Read the model definition and answer for the solid it produces. Units are mm, in the model's axes. A direction names the side the tool comes from. Give positions to 0.01 mm unless a question says otherwise; leave off trailing zeros. Order: outer loops, then holes, each group sorted by start corner. A loop starts at its lowest first (then second) coordinate and runs counter-clockwise, first axis right, second up. Notation, with made-up numbers: (-5.5, 68.25) -> (6.5, 68.25) arc R29 cw to (6.5, 93.25) -> close; hole circle Ø7 at (10, 75.5). An arc over 180 degrees is marked (long way). Answer as CSV lines item,"result". Start each with the question number.
1) A straight line is drawn through the part: L1, parallel to X at y = 212.5, z = 26. Find the intervals that lie inside material, in ascending order. Write a range as from..to.
2) Find section A-A (x = 60.5). Determine the outline of the cut face in (y, z).
3) Find section C-C (z = 13.5). Determine the outline of the cut face in (x, y).
4) For faces 1 (the face through (490, 252, 25)), 2 (the face through (247, 500, 25)), determine the directions among +Z, -Z, +X, -X, +Y, -Y from which every point of the face is accessible in a straight line to the end or side of a thin tool.
5) The mould has two halves that part along Y. Classify faces 3 (the face through (253, 0, 25)), 4 (the face through (10, 258, 25)), 5 (the face through (0, 252, 25)): +Y half, -Y half, draft (parallel to the pull), parting line (faces both ways), or undercut.
```python
from build123d import *

# Parameters (mm, degrees)
SALIENTE_EXTRUIR1_DEPTH = 50


with BuildPart() as part:
    # Croquis2 → Saliente-Extruir1 (new body)
    with BuildSketch(Plane.XY):
        with BuildLine():
            Line((0, 10), (0, 500))
            Line((0, 500), (500, 500))
            Line((500, 500), (500, 10))
            ThreePointArc((500, 10), (497.071067812, 2.928932188), (490, 0))
            Line((490, 0), (10, 0))
            ThreePointArc((10, 0), (2.928932188, 2.928932188), (0, 10))
        make_face()
        with BuildLine():
            Line((10, 490), (10, 20))
            ThreePointArc((10, 20), (12.928932188, 12.928932188), (20, 10))
            Line((20, 10), (480, 10))
            ThreePointArc((480, 10), (487.071067812, 12.928932188), (490, 20))
            Line((490, 20), (490, 490))
            Line((490, 490), (10, 490))
        make_face(mode=Mode.SUBTRACT)
    extrude(amount=SALIENTE_EXTRUIR1_DEPTH)


solid = part.part
```
Findings below:
1,L1,"0..10, 490..500"
2,outline,"(0, 0) -> (10, 0) -> (10, 50) -> (0, 50) -> close; (490, 0) -> (500, 0) -> (500, 50) -> (490, 50) -> close"
3,outline,"(0, 10) arc R10 ccw to (10, 0) -> (490, 0) arc R10 ccw to (500, 10) -> (500, 500) -> (0, 500) -> close; hole (10, 20) arc R10 ccw to (20, 10) -> (480, 10) arc R10 ccw to (490, 20) -> (490, 490) -> (10, 490) -> close"
4,face 1,"+Z, -Z"
4,face 2,"+Z, -Z, +X, -X, +Y"
5,face 3,"-Y half"
5,face 4,"undercut"
5,face 5,"draft"
